For this review, take the finished solid that the model builds, in its own axes (mm). Face numbers are marked on the shaded views. A direction names the side the tool comes from. Coordinates: 2 decimals unless noted, no trailing zeros. Order: outer loops, then holes, each group sorted by start corner. A loop starts at its lowest first (then second) coordinate and runs counter-clockwise, first axis right, second up. Notation, with made-up numbers: (-10.5, -20) -> (29.5, -20) arc R21 cw to (29.5, -7) -> close; hole circle Ø2 at (-26.5, -10.5). An arc over 180 degrees is marked (long way). Write item = value, one per line. Start each with the question number.
1) Consider section A-A on x = -4.5. Give the boundary of the cut face in (y, z).
2) Insertion check: pin 1 Ø8 at (x, z) = (73, 7) entering from -Y; pin 2 Ø3 at (x, z) = (33.5, -1) entering from +Y; pin 3 Ø5 at (x, y) = (28.5, -2) entering from -Z. Each pin has a flat end and moves straight along its axis. Give the tip position at first contact, or say it passes through.
3) Wall thickness on probe 1 along Z at (x, y) = (79.5, 0); probe 2 along X at (y, z) = (4.5, -7.5); probe 3 along Z at (x, y) = (51, -0.5): over which ranges is each line inside the solid? List them lowest first. Write a range as [from, to].
4) Consider section B-B on x = 7. Give the boundary of the cut face in (y, z).
5) Machinability: for the marked faces 1 and 2, which of the approach directions +Z, -Z, +X, -X, +Y, -Y give a long, thin tool a straight path to every point of the face, cutting with its end or side? Answer none if there is none.
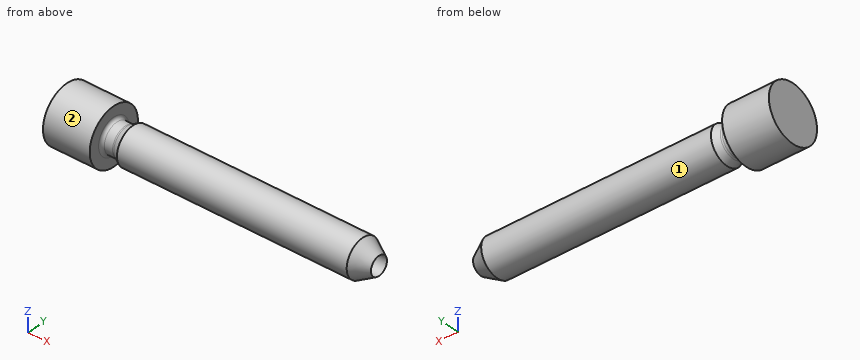
Autodesk Inventor part; units mm, degrees
ref_plane "YZ Plane" through (0, 0, 0) normal (1, 0, 0) x (0, 1, 0)
ref_plane "XZ Plane" through (0, 0, 0) normal (0, 1, 0) x (-1, 0, 0)
ref_plane "XY Plane" through (0, 0, 0) normal (0, 0, 1) x (1, 0, 0)
sketch "Skizze1" plane through (0, 0, 0) normal (0, 0, 1) x (1, 0, 0)
  line L0 (-35, 0) -> (105, 0)
  line L1 (0, -1.8) -> (0, 10.8)
  line L2 (0, 0) -> (65, 0)
  line L3 (85, 0) -> (85, 3)
  line L4 (79.8038, 6) -> (6.1517, 6)
  line L5 (0, 6) -> (0, 0)
  line L6 (0, 0) -> (-15, 0)
  line L7 (-15, 0) -> (-15, 9)
  line L8 (-15, 9) -> (0, 9)
  line L9 (0, 9) -> (0, 0)
  line L10 (85, 0) -> (65, 0)
  line L11 (85, 3) -> (85, 0)
  line L12 (85, 3) -> (79.8038, 6)
  line L13 (0, 0) -> (3.9, 0)
  line L14 (3.9, 0) -> (3.9, 4.7)
  line L15 (3.9, 4.7) -> (0, 4.7)
  line L16 (0, 4.7) -> (0, 0)
  line L17 (3.9, 4.7) -> (6.1517, 6)
  point P0 (85, 1.5)
  point P1 (0, 4.7)
  dimension "d2" = 9
  dimension "d3" = 100
  dimension "d7" = 30
  dimension "d8" = 12
  dimension "d10" = 6
  dimension "d11" = 85
  dimension "d12" = 9.4
  dimension "d13" = 3.9
  dimension "d17" = 30
revolve "Umdrehung1" add sketch "Skizze1" angle 360 about axis through (-10, 0, 0) along (1, 0, 0)
sketch "Skizze2" plane through (85, 0, 0) normal (1, 0, 0) x (0, 0, -1)
  point P0 (0, 0)
  point P1 (0, 0)
hole "Bohrung1" at (85, 0, 0) direction (-1, 0, 0) diameter 6 depth 20 tip angle 118
fillet "Rundung1" radius 1 1 edges at (0, -4.7, 0)
fillet "Rundung2" radius 1 1 edges at (3.9, -4.7, 0)
thread "Gewinde1"
sketch "Skizze3" plane through (-15, 0, 0) normal (-1, 0, 0) x (0, 0, 1)
  point P0 (0, 0)
properties part number "2.3_Druckschraube" material "1.0038 S235JR"
Answer sheet:
q1.outline = circle Ø18 at (0, 0)
q2.pin_1 = -5.2
q2.pin_2 = 6
q2.pin_3 = -6
q3.probe_1 = [-6, -3], [3, 6]
q3.probe_2 = [-15, 0]
q3.probe_3 = [-5.98, 5.98]
q4.outline = circle Ø12 at (0, 0)
q5.face_1 = +X
q5.face_2 = +X, -X
